Input: part model. Units: mm. Frame: model coordinates. Face numbers are marked on the shaded views. A direction names the side the tool comes from. Give positions to 0.01 mm unless a question says otherwise; leave off trailing zeros. Loops run counter-clockwise (first coordinate to the right, second up) from the corner with the lowest first, then second, coordinate; pieces in that order, holes last. Notation, with made-up numbers: (71, 72) - (126, 72) arc R12 ccw to (126, 84) - close; hole circle Ø7 at (-2, 7.5). An arc over 180 degrees is marked (long way). Answer as a JSON object with one key per item and string values. Group by question number.
(1) Material intervals for L1, parallel to X at y = 2.65, z = 3.75; L2, parallel to Y at x = 9, z = 1.55; L3, parallel to X at y = 1.4, z = 3.5, sorted ascending.
(2) Pin query (flat end, axial travel): P1, Ø1, axis at x = 12, z = 3.5, coming from the +Y side; P2, Ø1.8, axis at x = 10, y = 2, coming from the +Z side. Return the tip coordinate at first contact, or that it passes through.
(3) Section query C-C (z = 8.5). Return loops of the section in (x, y).
(4) Access query for the marked faces 4, 5 and 6. Directions: +Z, -Z, +X, -X, +Y, -Y. A direction counts if a zero-diameter tool reaches every point of the face in a straight line with its end or side. Return the directions, or none.
(5) Mould query, pull axis Y, two halves, no side actions, for the marked faces 1, 2 and 3. Classes: +Y half, -Y half, draft (parallel to the pull), parting line (faces both ways), or undercut.
(6) Section query D-D (z = 1.5). Return loops of the section in (x, y).
(7) Section query A-A (z = 4.25). Return loops of the section in (x, y).
(8) Section query B-B (x = 8). Return loops of the section in (y, z).
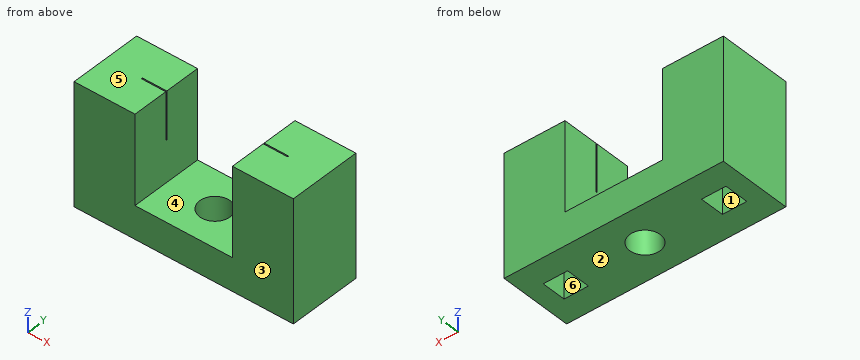
```python
from build123d import *

# Parameters (mm, degrees)
BOSS_EXTRUDE1_DEPTH = 6
SKETCH3_R           = 1.25
CUT_EXTRUDE1_DEPTH  = 2.7
SKETCH4_W           = 3.9
SKETCH4_H           = 0.1
CUT_EXTRUDE2_DEPTH  = 2
SKETCH5_W           = 2
SKETCH5_H           = 2
CUT_EXTRUDE3_DEPTH  = 8


with BuildPart() as part:
    # Sketch2 → Boss-Extrude1 (new body)
    with BuildSketch(Plane(origin=(0, 0, 0), x_dir=(1, 0, 0), z_dir=(0, 1, 0))):
        Polygon((0, 0), (18, 0), (18, -10), (13, -10), (13, -2.7), (5, -2.7), (5, -10), (0, -10), align=None)
    extrude(amount=BOSS_EXTRUDE1_DEPTH)

    # Sketch3 → Cut-Extrude1 (cut)
    with BuildSketch(Plane.XY.offset(2.7)):
        with Locations((9, 3)):
            Circle(SKETCH3_R)
    extrude(amount=-CUT_EXTRUDE1_DEPTH, mode=Mode.SUBTRACT)

    # Sketch4 → Cut-Extrude2 (cut)
    with BuildSketch(Plane(origin=(5, 0, 0), x_dir=(0, 0, -1), z_dir=(1, 0, 0))):
        with Locations((-8.05, 3)):
            Rectangle(SKETCH4_W, SKETCH4_H)
    cut_extrude2 = extrude(amount=-CUT_EXTRUDE2_DEPTH, mode=Mode.SUBTRACT)

    # Mirror1: Cut-Extrude2 across plane
    add(cut_extrude2.mirror(Plane(origin=(9, 0, 0), x_dir=(0, 0, 1), z_dir=(1, 0, 0))), mode=Mode.SUBTRACT)

    # Sketch5 → Cut-Extrude3 (cut)
    with BuildSketch(Plane(origin=(0, 0, 0), x_dir=(-1, 0, 0), z_dir=(0, 0, -1))):
        with Locations((-2.5, 3)):
            Rectangle(SKETCH5_W, SKETCH5_H)
    cut_extrude3 = extrude(amount=-CUT_EXTRUDE3_DEPTH, mode=Mode.SUBTRACT)

    # Mirror2: Cut-Extrude3 across plane
    add(cut_extrude3.mirror(Plane(origin=(9, 0, 0), x_dir=(0, 0, 1), z_dir=(1, 0, 0))), mode=Mode.SUBTRACT)


solid = part.part
```
Recorded:
{
 "1": {"L1": "x = 0 to 1.5, 3.5 to 5, 13 to 14.5, 16.5 to 18", "L2": "y = 0 to 1.75, 4.25 to 6", "L3": "x = 0 to 5, 13 to 18"},
 "2": {"P1": "passes through", "P2": "stops at z = 2.7"},
 "3": {"outline": "(0, 0) - (5, 0) - (5, 2.95) - (3, 2.95) - (3, 3.05) - (5, 3.05) - (5, 6) - (0, 6) - close; (13, 0) - (18, 0) - (18, 6) - (13, 6) - (13, 3.05) - (15, 3.05) - (15, 2.95) - (13, 2.95) - close"},
 "4": {"face 4": "+Z, +Y, -Y", "face 5": "+Z, +X, -X, +Y, -Y", "face 6": "-Z"},
 "5": {"face 1": "undercut", "face 2": "draft", "face 3": "-Y half"},
 "6": {"outline": "(0, 0) - (18, 0) - (18, 6) - (0, 6) - close; hole (1.5, 2) - (3.5, 2) - (3.5, 4) - (1.5, 4) - close; hole circle Ø2.5 at (9, 3); hole (14.5, 2) - (16.5, 2) - (16.5, 4) - (14.5, 4) - close"},
 "7": {"outline": "(0, 0) - (5, 0) - (5, 6) - (0, 6) - close; (13, 0) - (18, 0) - (18, 6) - (13, 6) - close; hole (1.5, 2) - (3.5, 2) - (3.5, 4) - (1.5, 4) - close; hole (14.5, 2) - (16.5, 2) - (16.5, 4) - (14.5, 4) - close"},
 "8": {"outline": "(0, 0) - (2.25, 0) - (2.25, 2.7) - (0, 2.7) - close; (3.75, 0) - (6, 0) - (6, 2.7) - (3.75, 2.7) - close"}
}
